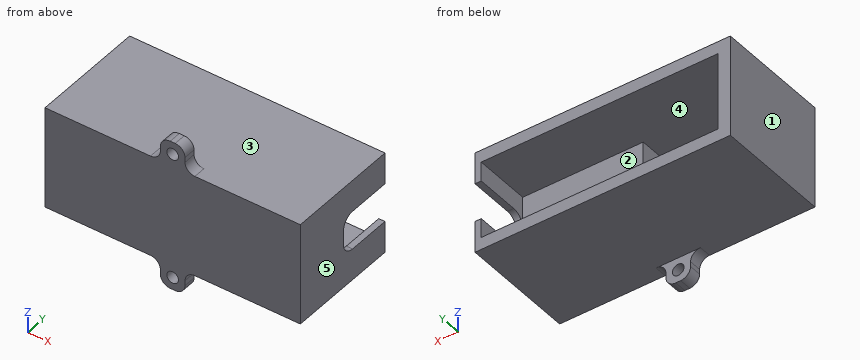
Autodesk Inventor part; units mm, degrees
ref_plane "Work Plane1" through (0, 0, 10) normal (0, 0, 1) x (1, 0, 0)
ref_plane "YZ Plane" through (0, 0, 0) normal (1, 0, 0) x (0, 1, 0)
ref_plane "XZ Plane" through (0, 0, 0) normal (0, 1, 0) x (-1, 0, 0)
sketch "Sketch1" plane through (0, 0, 0) normal (0, 0, 1) x (1, 0, 0)
  line L0 (0, 0) -> (32, 0)
  line L1 (32, 0) -> (32, 11.938)
  line L2 (32, 11.938) -> (0, 11.938)
  line L3 (0, 11.938) -> (0, 0)
  line L4 (0, 0) -> (-29, 0)
  line L5 (-29, 0) -> (-29, 11.938)
  line L6 (-29, 11.938) -> (0, 11.938)
  line L7 (0, 11.938) -> (0, 0)
  line L8 (32, 11.938) -> (-9, 11.938)
  line L9 (-9, 11.938) -> (-9, 23.938)
  line L10 (-9, 23.938) -> (32, 23.938)
  line L11 (32, 23.938) -> (32, 11.938)
  line L12 (32, 0) -> (33.6002, 0)
  line L13 (33.6002, 0) -> (33.6002, 23.938)
  line L14 (33.6002, 23.938) -> (32, 23.938)
  line L15 (32, 23.938) -> (32, 0)
  line L16 (33.6002, 0) -> (-29, 0)
  line L17 (-29, 0) -> (-29, -3.175)
  line L18 (-29, -3.175) -> (33.6002, -3.175)
  line L19 (33.6002, -3.175) -> (33.6002, 0)
  line L20 (-29, -3.175) -> (-32.175, -3.175)
  line L21 (-32.175, -3.175) -> (-32.175, 23.938)
  line L22 (-32.175, 23.938) -> (-29, 23.938)
  line L23 (-29, 23.938) -> (-29, -3.175)
  line L24 (-32.175, 23.938) -> (33.6002, 23.938)
  line L25 (33.6002, 23.938) -> (33.6002, 27.113)
  line L26 (33.6002, 27.113) -> (-32.175, 27.113)
  line L27 (-32.175, 27.113) -> (-32.175, 23.938)
  line L28 (0, 11.938) -> (0.9559, 11.938)
  line L29 (0.9559, 11.938) -> (0.9559, 0)
  line L30 (0.9559, 0) -> (0, 0)
  line L31 (0, 0) -> (0, 11.938)
  point P0 (0.9559, 0)
  dimension "d0" = 32
  dimension "d1" = 11.938
  dimension "d2" = 29
  dimension "d3" = 41
  dimension "d4" = 12
  dimension "d5" = 1.6002
  dimension "d7" = 3.175
  dimension "d8" = 3.175
  dimension "d9" = 3.175
extrude "Extrusion1" add sketch "Sketch1" along normal blind 20 contours L0 L12 L19 L18 L17 L4 | L29 L2 L1 L0 | L17 L20 L21 L22 L23 L5 | L1 L11 L14 L13 L12
sketch "Sketch2" plane through (0, 0, 20) normal (0, 0, 1) x (1, 0, 0)
  line L0 (-29, 23.938) -> (-32.175, 23.938)
  line L1 (-32.175, -3.175) -> (33.6002, -3.175)
  line L2 (-32.175, 23.938) -> (33.6002, 23.938)
  line L3 (33.6002, 23.938) -> (33.6002, -3.175)
  line L4 (33.6002, -3.175) -> (-32.175, -3.175)
  line L5 (-32.175, -3.175) -> (-32.175, 23.938)
  point P0 (0, 0)
  point P1 (-32.175, -3.175)
ref_plane "Work Plane1" through (0, 0, 10) normal (0, 0, 1) x (1, 0, 0)
extrude "Extrusion2" add sketch "Sketch2" along normal blind 3.175
mirror "Mirror1" about plane through (0, 0, 10) normal (0, 0, 1) of "Extrusion2"
sketch "Sketch3" plane through (33.6002, -3.175, 23.175) normal (1, 0, 0) x (0, 0, -1)
  line L0 (23.175, 15.113) -> (3.175, 15.113)
  line L1 (23.175, 27.113) -> (3.175, 27.113)
  line L2 (13.175, 15.113) -> (8.175, 15.113)
  line L3 (8.175, 15.113) -> (8.175, 27.113)
  line L4 (8.175, 27.113) -> (13.175, 27.113)
  line L5 (13.175, 27.113) -> (13.175, 15.113)
  line L6 (13.175, 27.113) -> (18.175, 27.113)
  line L7 (18.175, 27.113) -> (18.175, 15.113)
  line L8 (18.175, 15.113) -> (13.175, 15.113)
  line L9 (13.175, 15.113) -> (13.175, 27.113)
  point P0 (23.175, 3.175)
  dimension "d15" = 5
  dimension "d16" = 5
extrude "Extrusion3" cut sketch "Sketch3" against normal blind 3.175
fillet "Fillet1" radius 3.175 2 edges at (32.8001, 11.938, 5) (32.8001, 11.938, 15)
sketch "Sketch4" plane through (-32.175, -3.175, 23.175) normal (0, -1, 0) x (1, 0, 0)
  line L0 (65.7752, -8.175) -> (65.7752, 0)
  line L1 (65.7752, -26.35) -> (0, -26.35)
  line L2 (65.7752, 0) -> (0, 0)
  line L3 (0, 0) -> (0, -26.35)
  line L4 (0, -26.35) -> (65.7752, -26.35)
  line L5 (65.7752, -26.35) -> (65.7752, 0)
  line L6 (32.8876, 0) -> (36.0626, 0)
  line L7 (36.0626, 0) -> (36.0626, 6.35)
  line L8 (36.0626, 6.35) -> (32.8876, 6.35)
  line L9 (32.8876, 6.35) -> (32.8876, 0)
  line L10 (32.8876, 6.35) -> (29.7126, 6.35)
  line L11 (29.7126, 6.35) -> (29.7126, 0)
  line L12 (29.7126, 0) -> (32.8876, 0)
  line L13 (32.8876, 0) -> (32.8876, 6.35)
  circle A0 centre (32.8876, 3.175) radius 1.5
  line L14 (65.7752, -13.175) -> (55.6443, -13.175)
  line L15 (36.0626, -26.35) -> (36.0626, -32.7)
  line L16 (36.0626, -32.7) -> (32.8876, -32.7)
  line L17 (32.8876, -32.7) -> (29.7126, -32.7)
  line L18 (29.7126, -32.7) -> (29.7126, -26.35)
  circle A1 centre (32.8876, -29.525) radius 1.5
  point P0 (32.175, -23.175)
  dimension "d20" = 3.175
  dimension "d21" = 6.35
  dimension "d22" = 3.175
  dimension "d23" = 3
extrude "Extrusion4" add sketch "Sketch4" against normal blind 3.175 contours L2 L9 A0 L8 L7 | L2 L11 L10 L9 A0 | L15 L16 L17 L18 L1
fillet "Fillet2" radius 2.54 8 edges at (-2.4624, -1.5875, 23.175) (-2.4624, -1.5875, 29.525) (3.8876, -1.5875, 29.525) (3.8876, -1.5875, 23.175) (-2.4624, -1.5875, -9.525) (3.8876, -1.5875, -9.525) (3.8876, -1.5875, -3.175) (-2.4624, -1.5875, -3.175)
sketch "Sketch5" plane through (-29, 23.938, 20) normal (0, 1, 0) x (1, 0, 0)
  line L0 (62.6002, 5) -> (61, 5)
  line L1 (61, 5) -> (61, 0)
  line L2 (61, 0) -> (0, 0)
  line L3 (0, 20) -> (0, 0)
  line L4 (61, 20) -> (0, 20)
  line L5 (61, 20) -> (61, 15)
  line L6 (61, 15) -> (62.6002, 15)
  line L7 (62.6002, 23.175) -> (62.6002, 15)
  line L8 (62.6002, 23.175) -> (-3.175, 23.175)
  line L9 (-3.175, 23.175) -> (-3.175, -3.175)
  line L10 (62.6002, -3.175) -> (-3.175, -3.175)
  line L11 (62.6002, 5) -> (62.6002, -3.175)
  point P0 (29, 20)
extrude "Extrusion5" add sketch "Sketch5" along normal blind 2.54
properties part number "RadioMount" material "Rubber, Silicone"
Verification items for the finished model (mm, model axes). Face numbers are marked on the shaded views. A direction names the side the tool comes from. Round coordinates to 2 decimals unless told otherwise and drop trailing zeros. Write each loop counter-clockwise with the first axis right and the second up, starting at its lowest first coordinate (ties: lowest second). Pieces come first, ordered by that corner, then holes.
1. Access from +Z, -Z, +X, -X, +Y, -Y to the whole of each face (thin tool, end or side, straight path). Record for the marked faces 4 and 5.
2. Draft check along X on the marked faces 1, 2 and 3. Enter one of: +X half, -X half, draft (parallel to the pull), parting line (faces both ways), or undercut.
3. Section check B-B on x = -10.5. Enter the section's corners in (y, z) (3 decimals), plus the area to 3 significant figures.
4. Section check C-C on z = 2.5. Enter the section's corners in (x, y) (3 decimals), plus the area to 3 significant figures.
5. Scan lines: L1, parallel to Z at x = 30, y = 23 (3 decimals); L2, parallel to X at y = 8.5, z = 17 (3 decimals); L3, parallel to X at y = -2.4, z = 26.35. Record each from-to range of solid material in increasing order.
6. Gauge pin test, flat ends, axial feed: P1, Ø15, axis at x = -2, y = 15.5, coming from the -Z side (3 decimals); P2, Ø3, axis at x = -5.5, y = 11, coming from the +Z side (3 decimals); P3, Ø16, axis at x = 16, z = 10, coming from the +Y side; P4, Ø10, axis at x = 9, z = 0.5, coming from the +Y side. Record the tip position at first contact, or that the pin passes through.
7. Section check D-D on y = 20.5. Enter the section's corners in (x, z) (3 decimals).
8. Section check A-A on y = 8. Enter the section's corners in (x, z) (3 decimals).
Answer:
1. face 4: +Y
1. face 5: +Z, -Z, +X, +Y, -Y
2. face 1: -X half
2. face 2: undercut
2. face 3: draft
3. outline: (-3.175, -3.175) - (26.478, -3.175) - (26.478, 0) - (0, 0) - (0, 20) - (26.478, 20) - (26.478, 23.175) - (-3.175, 23.175) - close
3. area: 252 mm2
4. outline: (-32.175, -3.175) - (33.6, -3.175) - (33.6, 26.478) - (32, 26.478) - (32, 11.938) - (0.956, 11.938) - (0.956, 0) - (-29, 0) - (-29, 26.478) - (-32.175, 26.478) - close
4. area: 706 mm2
5. L1: z = -3.175 to 0, 20 to 23.175
5. L2: x = -32.175 to -29, 0.956 to 33.6
5. L3: x = -2.46 to -0.79, 2.21 to 3.89
6. P1: stops at z = -3.175
6. P2: stops at z = 23.175
6. P3: stops at y = 11.94
6. P4: stops at y = 26.48
7. outline: (-32.175, -3.175) - (33.6, -3.175) - (33.6, 5) - (32, 5) - (32, 0) - (-29, 0) - (-29, 20) - (32, 20) - (32, 15) - (33.6, 15) - (33.6, 23.175) - (-32.175, 23.175) - close
8. outline: (-32.175, -3.175) - (33.6, -3.175) - (33.6, 23.175) - (-32.175, 23.175) - close; hole (-29, 0) - (0.956, 0) - (0.956, 20) - (-29, 20) - close
